Verification items for this drawing (mm, ordinates from the low corner). A direction names the side the tool comes from. Coordinates: 2 decimals unless noted, no trailing zeros. Order: outer loops, then holes, each group sorted by start corner. A loop starts at its lowest first (then second) coordinate and runs counter-clockwise, first axis right, second up. Notation, with made-up numbers: M -2,3 L 2,3 A8 ccw 2,13 Z; hole C 31,74 d7. An arc over 180 degrees is marked long. Return JSON: item names as keys, results as strings. Group by question number.
1. Material ranges on line 1 along X through (y, z) = (6, 16.75); line 2 along X through (y, z) = (0.4, 18.8); line 3 along Y through (x, z) = (19.5, 6), recorded low to high.
2. Section check D-D, the plane z = 8. Record the cut outline in (x, y).
3. Gauge pin test, flat ends, axial feed: pin 1 (5.5 mm diameter, centred on x = 12.5, z = 17.5, fed in from +Y); pin 2 (2.5 mm diameter, centred on x = 16, y = 4, fed in from +Z); pin 3 (6 mm diameter, centred on x = 19, z = 4.5, fed in from +Y). Record the tip position at first contact, or that the pin passes through.
4. Mould release check, pull along Z, two halves, no side actions. Record for the marked faces 4, 5 and 6: +Z half, -Z half, draft (parallel to the pull), parting line (faces both ways), or undercut.
5. Set-up check for the marked faces 1, 2 and 3: record each of +Z, -Z, +X, -X, +Y, -Y from which the full face is reachable in a straight line by a thin tool's end or side.
6. Section check C-C, the plane x = 28. Record the cut outline in (y, z).
7. Section check A-A, the plane z = 2. Record the cut outline in (x, y).
8. Section check B-B, the plane y = 1.75. Record the cut outline in (x, z), plus the area to 3 significant figures.
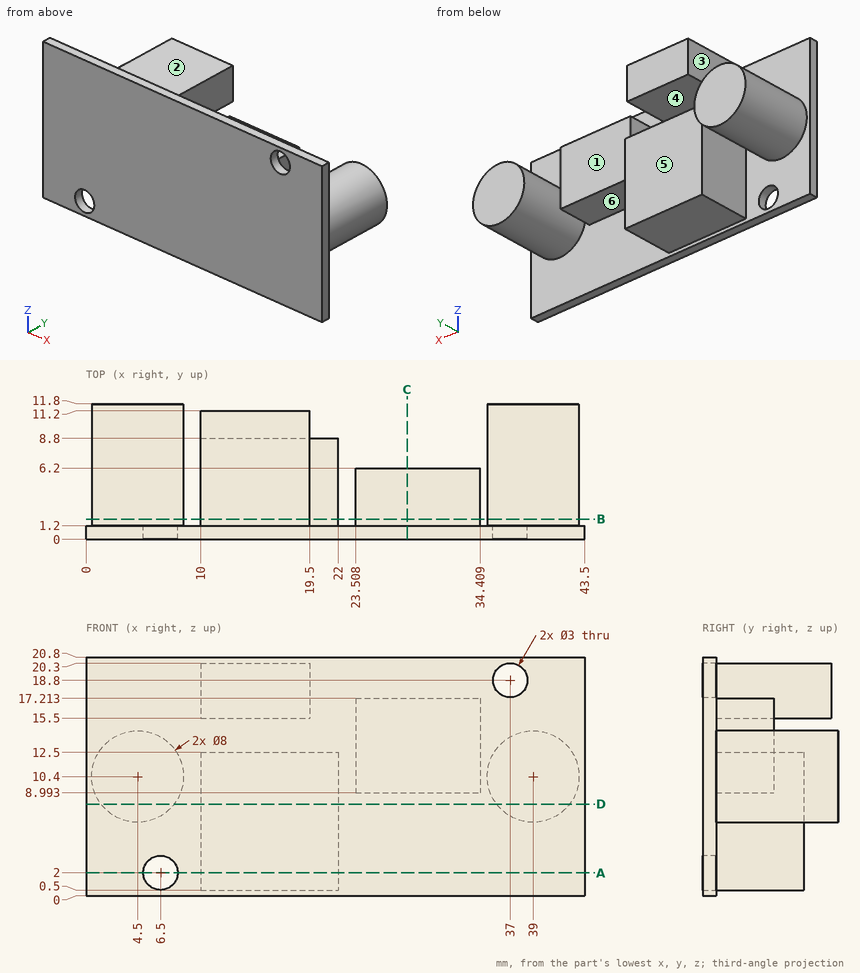
Answers follow:
{
 "1": {"line 1": "10 to 19.5, 23.51 to 34.41", "line 2": "0 to 35.5, 38.5 to 43.5", "line 3": "0 to 8.8"},
 "2": {"outline": "M 0,0 L 43.5,0 L 43.5,1.2 L 42.2,1.2 L 42.2,11.8 L 35.8,11.8 L 35.8,1.2 L 22,1.2 L 22,8.8 L 10,8.8 L 10,1.2 L 7.7,1.2 L 7.7,11.8 L 1.3,11.8 L 1.3,1.2 L 0,1.2 Z"},
 "3": {"pin 1": "y = 11.2", "pin 2": "z = 20.3", "pin 3": "y = 8.8"},
 "4": {"face 4": "undercut", "face 5": "draft", "face 6": "-Z half"},
 "5": {"face 1": "+Z, -Z, +Y", "face 2": "+Z, +X, -X, +Y", "face 3": "+Z, -Z, -X, +Y"},
 "6": {"outline": "M 0,0 L 1.2,0 L 1.2,8.99 L 6.2,8.99 L 6.2,17.21 L 1.2,17.21 L 1.2,20.8 L 0,20.8 Z"},
 "7": {"outline": "M 0,0 L 5,0 L 5,1.2 L 0,1.2 Z; M 8,0 L 43.5,0 L 43.5,1.2 L 22,1.2 L 22,8.8 L 10,8.8 L 10,1.2 L 8,1.2 Z"},
 "8": {"outline": "C 4.5,10.4 d8; M 10,0.5 L 22,0.5 L 22,12.5 L 10,12.5 Z; M 10,15.5 L 19.5,15.5 L 19.5,20.3 L 10,20.3 Z; M 23.51,8.99 L 34.41,8.99 L 34.41,17.21 L 23.51,17.21 Z; C 39,10.4 d8", "area": "380 mm^2"}
}
